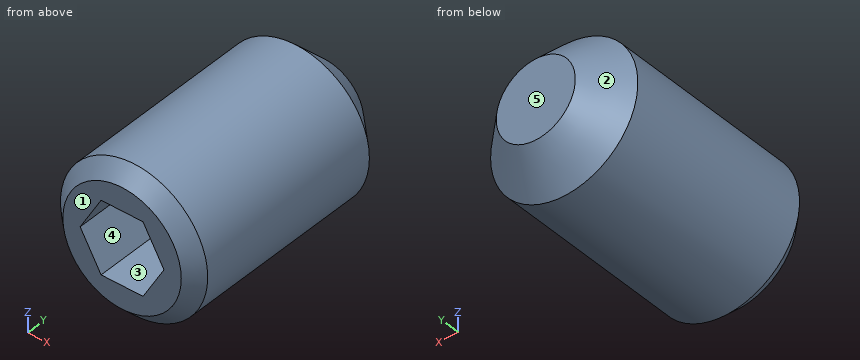
from build123d import *

# Parameters (mm, degrees)
CUT_EXTRUDE1_DEPTH = 2.54
CHAMFER1_SIZE      = 0.47244


with BuildPart() as part:
    # Sketch1 → Revolve1 (revolve)
    with BuildSketch(Plane(origin=(0, 0, 0), x_dir=(-1, 0, 0), z_dir=(0, 0, -1))):
        Polygon((-2.413, 0), (0, 0), (0, 7.9375), (-1.2954, 7.9375), (-2.413, 6.8199), align=None)
    revolve(axis=Axis((0, 0, 0), (0, 1, 0)))

    # Sketch2 → Cut-Extrude1 (cut)
    with BuildSketch(Plane.XZ):
        Polygon((-0.68704079, 1.189989555), (-1.37408158, 0), (-0.68704079, -1.189989555), (0.68704079, -1.189989555), (1.37408158, 0), (0.68704079, 1.189989555), align=None)
    extrude(amount=-CUT_EXTRUDE1_DEPTH, mode=Mode.SUBTRACT)

    # Chamfer1
    chamfer1_edges = [part.edges().sort_by_distance(p)[0] for p in [
        (-2.413, 0, 0),
    ]]
    chamfer(chamfer1_edges, length=CHAMFER1_SIZE)


solid = part.part
Design review of the part built by this model. Coordinates are the model's own, in mm. Face numbers are marked on the shaded views. A direction names the side the tool comes from. Round coordinates to 2 decimals unless told otherwise and drop trailing zeros. Loops run counter-clockwise (first coordinate to the right, second up) from the corner with the lowest first, then second, coordinate; pieces in that order, holes last. Notation, with made-up numbers: M 47.5,57 L 98.5,57 A10 cw 98.5,63 Z; hole C 89.5,36 d1. An arc over 180 degrees is marked long. Answer as a JSON object with one key per item and string values.
Item 1: We need section A-A on y = 1.75. Give the boundary of the cut face in (x, z), and give its area (3 significant figures).
Answer sheet:
{"outline": "C 0,0 d4.83; hole M -1.37,0 L -0.69,-1.19 L 0.69,-1.19 L 1.37,0 L 0.69,1.19 L -0.69,1.19 Z", "area": "13.4 mm^2"}
Item 2: We need section B-B on x = 0. Give the boundary of the cut face in (y, z).
Answer sheet:
{"outline": "M 0,-1.94 L 0.47,-2.41 L 6.82,-2.41 L 7.94,-1.3 L 7.94,1.3 L 6.82,2.41 L 0.47,2.41 L 0,1.94 L 0,1.19 L 2.54,1.19 L 2.54,-1.19 L 0,-1.19 Z"}
Item 3: The part is to be moulded in two halves that separate along Z. For the marked faces 1, 2 and 3, say which applies: pulls with the +Z half, pulls with the -Z half, needs draft (parallel to the pull), parting line crosses it, or undercut.
Answer sheet:
{"face 1": "needs draft", "face 2": "parting line crosses it", "face 3": "undercut"}
Item 4: Machinability: for the marked faces 4 and 5, which of the approach directions +Z, -Z, +X, -X, +Y, -Y give a long, thin tool a straight path to every point of the face, cutting with its end or side? Answer none if there is none.
Answer sheet:
{"face 4": "-Y", "face 5": "+Z, -Z, +X, -X, +Y"}
Item 5: Wall thickness on L1, parallel to Z at x = -0.05, y = 1.25; L2, parallel to Z at x = -2.1, y = 1; L3, parallel to Y at x = 0.25, z = -0.9: over which ranges is each line inside the solid? List them lowest first. Write a range as from..to.
Answer sheet:
{"L1": "z = -2.41..-1.19, 1.19..2.41", "L2": "z = -1.19..1.19", "L3": "y = 2.54..7.94"}
Item 6: We need section C-C on y = 6.5. Give the boundary of the cut face in (x, z).
Answer sheet:
{"outline": "C 0,0 d4.83"}
